Source: CAD feature listing. Evaluate the final solid. Frame: model axes, mm. A direction names the side the tool comes from. Give positions to 0.01 mm unless a question says otherwise; leave off trailing zeros. Loops run counter-clockwise (first coordinate to the right, second up) from the corner with the lowest first, then second, coordinate; pieces in that order, holes last.
from build123d import *

# Parameters (mm, degrees)
WHOLEBODY_DEPTH    = 280
UPPERCURVE_DEPTH   = 286.41198293
SKETCH6_W          = 32
SKETCH6_H          = 5
CUT_EXTRUDE5_DEPTH = 285.921480537
CUT_EXTRUDE6_DEPTH = 286.411983055
UPPERHOLE_DEPTH    = 289.81308838
CHAMFER1_SIZE      = 10
CUT_EXTRUDE8_DEPTH = 286.411982957
CUT_EXTRUDE9_DEPTH = 286.411982957


with BuildPart() as part:
    # Sketch1 → WholeBody (new body)
    with BuildSketch(Plane.XY):
        with BuildLine():
            Line((0, 0), (0, -36))
            Line((0, -36), (42, -36))
            Line((42, -36), (42, 0))
            ThreePointArc((42, 0), (21, 21), (0, 0))
        make_face()
    extrude(amount=-WHOLEBODY_DEPTH)

    # Sketch2 → UpperCurve (cut, through all)
    with BuildSketch(Plane(origin=(42, 0, 0), x_dir=(0, 0, -1), z_dir=(1, 0, 0))):
        with BuildLine():
            ThreePointArc((29, -36), (0.5, -7.5), (29, 21))
            Line((29, 21), (0, 21))
            Line((0, 21), (0, 0))
            Line((0, 0), (0, -36))
            Line((0, -36), (29, -36))
        make_face()
    extrude(amount=-UPPERCURVE_DEPTH, mode=Mode.SUBTRACT)

    # Sketch6 → Cut-Extrude5 (cut, through all)
    with BuildSketch(Plane(origin=(0, 0, -280), x_dir=(-1, 0, 0), z_dir=(0, 0, -1))):
        with BuildLine():
            Line((-37, 0), (-37, -31))
            Line((-37, -31), (-5, -31))
            Line((-5, -31), (-5, 0))
            ThreePointArc((-5, 0), (-21, 16), (-37, 0))
        make_face()
        with Locations((-21, -33.5)):
            Rectangle(SKETCH6_W, SKETCH6_H)
    extrude(amount=-CUT_EXTRUDE5_DEPTH, mode=Mode.SUBTRACT)

    # Sketch8 → Cut-Extrude6 (cut, through all)
    with BuildSketch(Plane.ZY):
        Polygon((-263.367084443, 0), (-226.082527774, 21), (-280, 21), (-280, 0), align=None)
        with BuildLine():
            Line((-270.565078665, -4.054168593), (-263.367084443, 0))
            Line((-263.367084443, 0), (-280, 0))
            Line((-280, 0), (-280, -20.196793601))
            ThreePointArc((-280, -20.196793601), (-277.468291323, -10.847969039), (-270.565078665, -4.054168593))
        make_face()
        with BuildLine():
            ThreePointArc((-265.552960254, -36), (-275.843932749, -30.902613162), (-280, -20.196793601))
            Line((-280, -20.196793601), (-280, -36))
            Line((-280, -36), (-265.552960254, -36))
        make_face()
    extrude(amount=-CUT_EXTRUDE6_DEPTH, mode=Mode.SUBTRACT)

    # Sketch9 → UpperHole (cut, through all)
    with BuildSketch(Plane.XZ.offset(36)):
        Polygon((5, -0.5), (5, -57.942137899), (37, -57.942137899), (37, -29), (37, 4.098042087), (5, 4.098042087), align=None)
    extrude(amount=-UPPERHOLE_DEPTH, mode=Mode.SUBTRACT)

    # Chamfer1
    # the kernel refuses this chamfer: 10 mm, written as the material it takes off along each edge
    with BuildSketch(Plane(origin=(21, 0, -57.942137899), x_dir=(0.86749005683434, -0.49745452183446237, 0), z_dir=(-0.49745452183446237, -0.86749005683434, 0))) as chamfer1_piece_1_section:
        Polygon((21, -CHAMFER1_SIZE), (21 - CHAMFER1_SIZE, 0), (21, 0), align=None)
    chamfer1_piece_1 = revolve(axis=Axis((21, 0, -57.942137899), (0, 0, 1)), revolution_arc=239.663469858, mode=Mode.PRIVATE)
    chamfer1_piece_1 = split(chamfer1_piece_1, bisect_by=Plane(origin=(5, 16.096053983, -62.846083916), z_dir=(1, 0, 0)), keep=Keep.TOP, mode=Mode.PRIVATE)
    chamfer1_piece_1 = split(chamfer1_piece_1, bisect_by=Plane(origin=(37, 16.096053983, -62.846083916), z_dir=(-1, 0, 0)), keep=Keep.TOP, mode=Mode.PRIVATE)
    add(chamfer1_piece_1, mode=Mode.SUBTRACT)

    # Sketch11 → Cut-Extrude8 (cut, through all)
    with BuildSketch(Plane.ZY):
        with BuildLine():
            Line((-9.843331647, 13.601470509), (-14.201102996, 13.601470509))
            ThreePointArc((-14.201102996, 13.601470509), (-9.729411408, 12.545964589), (-6.20169921, 9.602265378))
            ThreePointArc((-6.20169921, 9.602265378), (-7.927428506, 11.688453055), (-9.843331647, 13.601470509))
        make_face()
    extrude(amount=-CUT_EXTRUDE8_DEPTH, mode=Mode.SUBTRACT)

    # Sketch12 → Cut-Extrude9 (cut, through all)
    with BuildSketch(Plane.ZY):
        with BuildLine():
            Line((-204.781024531, -15.957949817), (-95.140934308, -15.957949817))
            ThreePointArc((-95.140934308, -15.957949817), (-90.128815898, -20.970068227), (-95.140934308, -25.982186638))
            Line((-95.140934308, -25.982186638), (-204.781024531, -25.982186638))
            ThreePointArc((-204.781024531, -25.982186638), (-209.793142941, -20.970068227), (-204.781024531, -15.957949817))
        make_face()
    extrude(amount=-CUT_EXTRUDE9_DEPTH, mode=Mode.SUBTRACT)


solid = part.part
1) Cut plane B-B (z = -42). Return loops of the section in (x, y), and give its area (3 significant figures).
Checks:
outline: (0, -36) - (5, -36) - (5, 13.6) arc R21 ccw to (0, 0) - close; (37, -36) - (42, -36) - (42, 0) arc R21 ccw to (37, 13.6) - close
area: 453 mm2
2) Cut plane D-D (x = 21). Return loops of the section in (y, z), and give its area (3 significant figures).
Checks:
outline: (16, -234.96) - (21, -226.08) - (21, -67.94) - (16, -62.94) - close
area: 825 mm2
3) Ray query, probe 1 along X at (y, z) = (-8.5, -16); probe 2 along Y at (x, z) = (20, -210); probe 3 along Z at (x, y) = (38, -19). Return the intervals inside material, ascending.
Checks:
probe 1: x = 0 to 5, 37 to 42
probe 2: y = 15.97 to 20.98
probe 3: z = -279.96 to -209.39, -90.53 to -2.92
4) Pull-direction query (X, two-part tool) for faces 1 (the cylindrical face through (39.465, -31.023, -275.732)), 2 (the flat face through (5, -12, -138)), 3 (the cylindrical face through (21, 21, -131)), 4 (the conical face through (21.357, 16.239, -63.185)); classes: released by +X, released by -X, zero draft, split by the parting line, or undercut.
Checks:
face 1: zero draft
face 2: undercut
face 3: split by the parting line
face 4: undercut
5) Reachability of faces 5 (the cylindrical face through (39.47, -21.08, -209.79)), 6 (the cylindrical face through (39.53, -20.64, -3.71)) from +Z, -Z, +X, -X, +Y, -Y: full face, straight path, thin tool, end or side. Return the list, or none.
Checks:
face 5: +X, -X
face 6: +Z, +X, -X
6) Cut plane A-A (z = -106). Return loops of the section in (x, y), and give its area (3 significant figures).
Checks:
outline: (0, -36) - (5, -36) - (5, -25.98) - (0, -25.98) - close; (0, -15.96) - (5, -15.96) - (5, 0) arc R16 cw to (37, 0) - (37, -15.96) - (42, -15.96) - (42, 0) arc R21 ccw to (0, 0) - close; (37, -36) - (42, -36) - (42, -25.98) - (37, -25.98) - close
area: 550 mm2
7) Contact query for flat-ended pins moving along their axis: P1, Ø4, axis at x = 2, z = -129, coming from the +Y side; P2, Ø4, axis at x = 39, z = -126.5, coming from the +Y side; P3, Ø1, axis at y = 3.5, z = -47, coming from the -X side; P4, Ø25, axis at y = -6, z = -202, coming from the -X side. Output: stop coordinate, or through.
Checks:
P1: stops at y = 12.33
P2: stops at y = 13.6
P3: stops at x = 0.22
P4: stops at x = 0
8) Cut plane C-C (y = -6.5). Return loops of the section in (x, z).
Checks:
outline: (0, -273.95) - (5, -273.95) - (5, -0.52) - (0, -0.52) - close; (37, -273.95) - (42, -273.95) - (42, -0.52) - (37, -0.52) - close
